Autodesk Fusion 360 part; units mm, degrees
sketch "スケッチ1" plane through (0, 0, 0) normal (0, 0, 1) x (1, 0, 0)
  line L0 (0, 0) -> (33, 0)
  line L1 (33, 0) -> (33, 18)
  line L2 (33, 18) -> (0, 18)
  line L3 (0, 18) -> (0, 0)
  dimension "d1" = 33
  dimension "d2" = 18
extrude "押し出し1" add sketch "スケッチ1" along normal blind 4
sketch "スケッチ2" plane through (0, 0, 4) normal (0, 0, 1) x (-1, 0, 0)
  line L0 (0, -18) -> (0, 0)
  line L1 (0, 0) -> (-33, 0)
  line L2 (-33, 0) -> (-33, -18)
  line L3 (-33, -18) -> (0, -18)
  line L4 (-33, -18) -> (-28, -18)
  line L5 (-28, -18) -> (-28, 0)
  line L6 (-28, 0) -> (-33, 0)
  line L7 (-33, 0) -> (-33, -18)
  line L8 (-28, -12.75) -> (-33, -12.75)
  line L9 (-33, -12.75) -> (-33, -5.25)
  line L10 (-33, -5.25) -> (-28, -5.25)
  line L11 (-28, -5.25) -> (-28, -12.75)
  line L12 (-31.75, -9) -> (-34.25, -9) construction
  line L13 (-34.25, -9) -> (-31.75, -9) construction
  line L14 (0, 0) -> (-28, 0)
  line L15 (-28, 0) -> (-28, -2.5)
  line L16 (-28, -2.5) -> (0, -2.5)
  line L17 (0, -2.5) -> (0, 0)
  line L18 (0, -18) -> (-28, -18)
  line L19 (-28, -18) -> (-28, -15.5)
  line L20 (-28, -15.5) -> (0, -15.5)
  line L21 (0, -15.5) -> (0, -18)
  dimension "d5" = 5
  dimension "d6" = 18
  dimension "d7" = 5
  dimension "d8" = 7.5
  dimension "d11" = 2.5
  dimension "d12" = 2.5
extrude "押し出し2" cut sketch "スケッチ2" against normal blind 2.5 contours L0 L3 L5 L18 L19 L20 L21 | L2 L3 L4 L5 L7 L8 L19 | L0 L1 L5 L14 L15 L16 L17 | L1 L2 L5 L6 L7 L10 L15
sketch "スケッチ3" plane through (33, 0, 0) normal (1, 0, 0) x (0, 1, 0)
  line L0 (5.25, 4) -> (5.25, 1.5)
  line L1 (5.25, 1.5) -> (0, 1.5)
  line L2 (0, 1.5) -> (0, 0)
  line L3 (0, 0) -> (18, 0)
  line L4 (18, 0) -> (18, 1.5)
  line L5 (18, 1.5) -> (12.75, 1.5)
  line L6 (12.75, 1.5) -> (12.75, 4)
  line L7 (12.75, 4) -> (5.25, 4)
  line L8 (12.75, 1.5) -> (5.25, 1.5)
  line L9 (5.25, 1.5) -> (5.25, 4)
  line L10 (5.25, 4) -> (12.75, 4)
  line L11 (12.75, 4) -> (12.75, 1.5)
extrude "押し出し3" add sketch "スケッチ3" along normal blind 0.6 contours L0 L6 L7 L8 L9 L10 L11
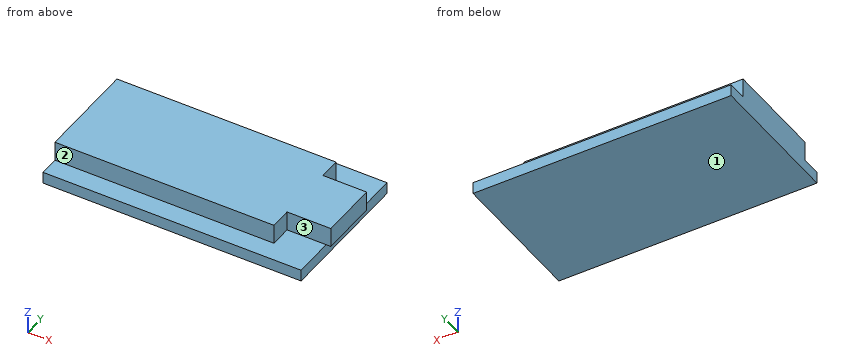
Could you check a few things on this model? Use its own coordinates, in mm. Face numbers are marked on the shaded views. A direction names the side the tool comes from. Give positions to 0.01 mm unless a question says otherwise; leave off trailing zeros. Loops run counter-clockwise (first coordinate to the right, second up) from the corner with the lowest first, then second, coordinate; pieces in that order, holes last. Notation, with made-up numbers: (-35, 7) - (14, 7) arc R15 ccw to (14, 30) - close; hole circle Ø5 at (56.25, -38). An arc over 180 degrees is marked (long way). Use one line per item in the form item = value.
1. I need wall thicknesses on probe 1 along X at (y, z) = (3.25, 1.9); probe 2 along Y at (x, z) = (22, 2.7); probe 3 along X at (y, z) = (14.75, 0.6). Which ranges of each line are inside material? Lowest first, please.
Response values:
probe_1 = 0 to 28
probe_2 = 2.5 to 15.5
probe_3 = 0 to 33
2. I want a section at D-D (y = 1). Please give me the cut outline in (x, z).
Response values:
outline = (0, 0) - (33, 0) - (33, 1.5) - (0, 1.5) - close
3. I want a section at C-C (y = 3.5). Please give me the cut outline in (x, z).
Response values:
outline = (0, 0) - (33, 0) - (33, 1.5) - (28, 1.5) - (28, 4) - (0, 4) - close
4. On a 3-axis mill with a long thin cutter (end or side, diameter ignored), from which of +Z, -Z, +X, -X, +Y, -Y can I reach the whole of each face in a straight line? I mean the marked faces 1, 2 and 3. Say none if no direction works.
Response values:
face_1 = -Z, +X, -X, +Y, -Y
face_2 = +Z, +X, -X, -Y
face_3 = +Z, +X, -Y
5. I want a section at A-A (x = 17). Please give me the cut outline in (y, z), and give its area (3 significant figures).
Response values:
outline = (0, 0) - (18, 0) - (18, 1.5) - (15.5, 1.5) - (15.5, 4) - (2.5, 4) - (2.5, 1.5) - (0, 1.5) - close
area = 59.5 mm²
6. I'm going to push flat-ended pins straight in: pin 1 Ø2 at (x, z) = (18, 3) entering from -Y; pin 2 Ø1.2 at (x, z) = (32, 3) entering from +Y; pin 3 Ø2 at (y, z) = (14.5, 3.5) entering from +X. Where does each tip first touch, or does it pass through?
Response values:
pin_1 = 2.5
pin_2 = 12.75
pin_3 = 28
7. I want a section at B-B (z = 2.05). Please give me the cut outline in (x, y), and give its area (3 significant figures).
Response values:
outline = (0, 2.5) - (28, 2.5) - (28, 5.25) - (33.6, 5.25) - (33.6, 12.75) - (28, 12.75) - (28, 15.5) - (0, 15.5) - close
area = 406 mm²
